from build123d import *

# Parameters (mm, degrees)
F1_DEPTH = 79.375
F2_W     = 19.05
F2_H     = 98.425
F3_DEPTH = 31.75
F4_R     = 4.7625
F5_DEPTH = 49.2135
F6_R     = 4.7625
F7_DEPTH = 98.426


with BuildPart() as f1:
    # F0 (on Front) → F1 (new body)
    with BuildSketch(Plane.XZ):
        Polygon((-39.476471, 39.877854), (-39.476471, -58.547146), (-29.951471, -58.547146), (-29.951471, -4.572146), (1.798529, -4.572146), (1.798529, 4.952854), (-29.951471, 4.952854), (-29.951471, 30.352854), (1.798529, 30.352854), (1.798529, 39.877854), align=None)
    extrude(amount=F1_DEPTH)

    # F2 (on face) → F3 (join)
    with BuildSketch(Plane(origin=(-39.476471, 0, 0), x_dir=(0, -1, 0), z_dir=(-1, 0, 0))):
        with Locations((39.6875, -9.334646)):
            Rectangle(F2_W, F2_H)
    extrude(amount=F3_DEPTH)

    # F4 (on face) → F5 (cut, through all)
    with BuildSketch(Plane.XZ.offset(49.2125)):
        with Locations((-55.351471, 28.765354)):
            Circle(F4_R)
        with Locations((-55.351471, 3.365354)):
            Circle(F4_R)
        with Locations((-55.351471, -22.034646)):
            Circle(F4_R)
        with Locations((-55.351471, -47.434646)):
            Circle(F4_R)
    extrude(amount=-F5_DEPTH, mode=Mode.SUBTRACT)

    # F6 (on face) → F7 (cut, through all)
    with BuildSketch(Plane.XY.offset(39.877854)):
        with Locations((-14.076471, -15.875)):
            Circle(F6_R)
        with Locations((-14.076471, -41.275)):
            Circle(F6_R)
        with Locations((-14.076471, -66.675)):
            Circle(F6_R)
    extrude(amount=-F7_DEPTH, mode=Mode.SUBTRACT)


solid = f1.part
Design review of the part built by this model. Coordinates are the model's own, in mm. A direction names the side the tool comes from. Coordinates: 2 decimals unless noted, no trailing zeros. Order: outer loops, then holes, each group sorted by start corner. A loop starts at its lowest first (then second) coordinate and runs counter-clockwise, first axis right, second up. Notation, with made-up numbers: M -14,-30.5 L 44,-30.5 A22 cw 44,-21.5 Z; hole C -31,63.5 d9. An arc over 180 degrees is marked long. Use a Markdown table: item, result.
(1) Wall thickness on probe 1 along X at (y, z) = (-16, 1.5); probe 2 along Z at (x, y) = (-20.5, -16); probe 3 along X at (y, z) = (-41.5, 34.5): over which ranges is each line inside the solid? List them lowest first.
Worked answers:
| item | result |
|---|---|
| probe 1 | x = -39.48 to -18.84, -9.32 to 1.8 |
| probe 2 | z = -4.57 to 4.95, 30.35 to 39.88 |
| probe 3 | x = -71.23 to -18.83, -9.32 to 1.8 |
(2) For faces 1 (the flat face through (-39.476, -15, -9)), 2 (the flat face through (-7, -39, 4.953)), 3 (the flat face through (-71.226, -40, -9)), 4 (the flat face through (-29.951, -39, -32)), list the 3-axis set-ups (+Z, -Z, +X, -X, +Y, -Y) from which the entire face can be reached by the end or side of a thin tool; tool diameter is ignored.
Worked answers:
| item | result |
|---|---|
| face 1 | +Z, -Z, -X, +Y |
| face 2 | +X, +Y, -Y |
| face 3 | +Z, -Z, -X, +Y, -Y |
| face 4 | -Z, +X, +Y, -Y |
(3) Add section A-A (x = -24). Give the boundary of the cut face in (y, z) (3 decimals), then the cut area to 3 significant figures.
Worked answers:
| item | result |
|---|---|
| outline | M -79.375,-4.572 L 0,-4.572 L 0,4.953 L -79.375,4.953 Z; M -79.375,30.353 L 0,30.353 L 0,39.878 L -79.375,39.878 Z |
| area | 1,510 mm2 |
(4) For P1, Ø15, axis at y = -66.5, z = -13, coming from the -X side; P2, Ø4, axis at y = -65, z = 28, coming from the +X side; P3, Ø3, axis at x = -55.5, z = -36, coming from the -Y side, all flat-tipped, find the tip position at first contact; note any pin that passes through.
Worked answers:
| item | result |
|---|---|
| P1 | stops at x = -39.48 |
| P2 | stops at x = -29.95 |
| P3 | stops at y = -49.21 |
(5) Add section C-C (z = 26.5). Give the boundary of the cut face in (x, y) (1 decimal).
Worked answers:
| item | result |
|---|---|
| outline | M -71.2,-49.2 L -59.5,-49.2 L -59.5,-30.2 L -71.2,-30.2 Z; M -51.2,-49.2 L -39.5,-49.2 L -39.5,-79.4 L -30,-79.4 L -30,0 L -39.5,0 L -39.5,-30.2 L -51.2,-30.2 Z |
(6) Add section B-B (y = -42.5). Give the boundary of the cut face in (x, z) (1 decimal), then the cut area to 3 significant figures.
Worked answers:
| item | result |
|---|---|
| outline | M -71.2,-58.5 L -30,-58.5 L -30,-4.6 L -18.7,-4.6 L -18.7,5 L -30,5 L -30,30.4 L -18.7,30.4 L -18.7,39.9 L -71.2,39.9 Z; M -9.5,-4.6 L 1.8,-4.6 L 1.8,5 L -9.5,5 Z; M -9.5,30.4 L 1.8,30.4 L 1.8,39.9 L -9.5,39.9 Z; hole C -55.4,-47.4 d9.5; hole C -55.4,-22 d9.5; hole C -55.4,3.4 d9.5; hole C -55.4,28.8 d9.5 |
| area | 4,210 mm2 |
(7) Draft analysis for pull direction Y (two halves, no side actions). For faces 5 (the flat face through (-55, -30.162, -10)), 6 (the cylindrical face through (-18.834, -66.466, 0.257)), 7 (the flat face through (1.799, -39, 0)), state which applies: released by +Y, released by -Y, zero draft, split by the parting line, or undercut.
Worked answers:
| item | result |
|---|---|
| face 5 | released by +Y |
| face 6 | undercut |
| face 7 | zero draft |
(8) Add section D-D (y = -70). Give the boundary of the cut face in (x, z), then the cut area to 3 significant figures.
Worked answers:
| item | result |
|---|---|
| outline | M -39.48,-58.55 L -29.95,-58.55 L -29.95,-4.57 L -17.49,-4.57 L -17.49,4.95 L -29.95,4.95 L -29.95,30.35 L -17.49,30.35 L -17.49,39.88 L -39.48,39.88 Z; M -10.67,-4.57 L 1.8,-4.57 L 1.8,4.95 L -10.67,4.95 Z; M -10.67,30.35 L 1.8,30.35 L 1.8,39.88 L -10.67,39.88 Z |
| area | 1,410 mm2 |
